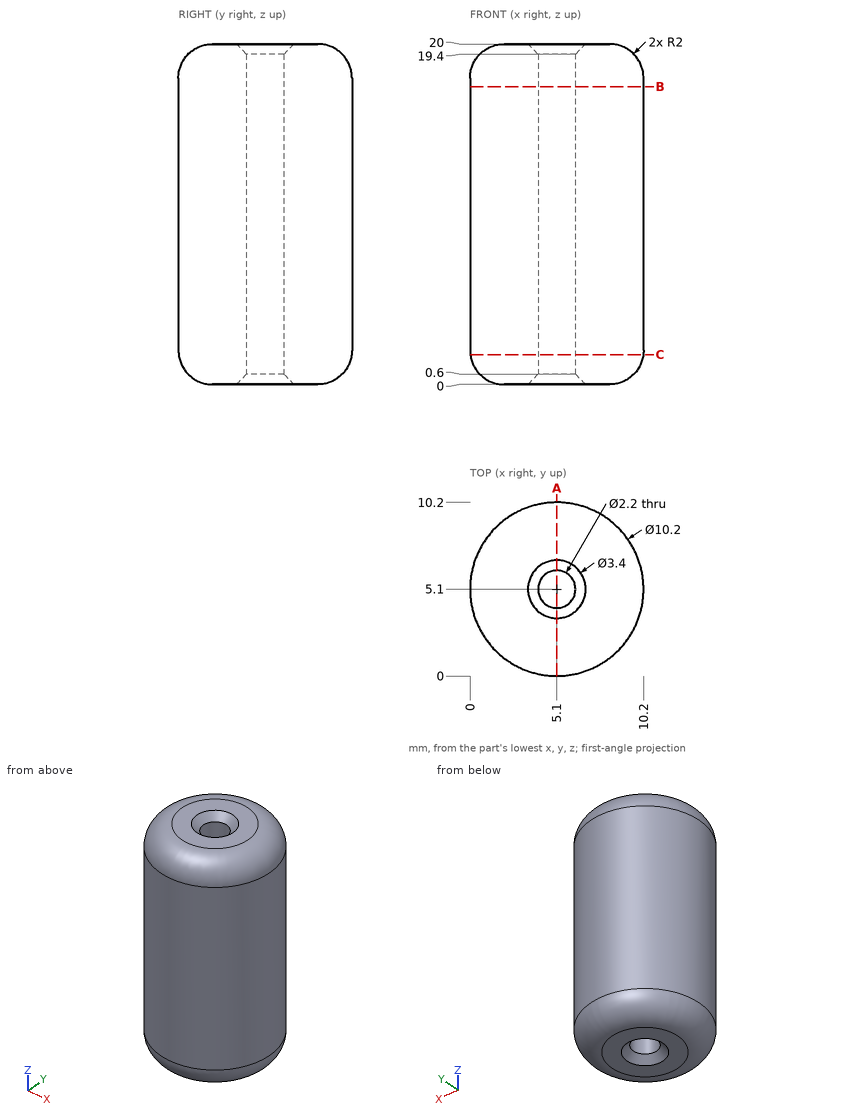
Input: dimensioned drawing with shaded views. Units: mm. Origin: part minimum x, y, z. Round coordinates to 2 decimals unless told otherwise and drop trailing zeros. Order: outer loops, then holes, each group sorted by start corner. A loop starts at its lowest first (then second) coordinate and runs counter-clockwise, first axis right, second up.
1. Pin query (flat end, axial travel): P1, Ø2.5, axis at x = 5.1, y = 5.1, coming from the +Z side; P2, Ø2, axis at x = 5, y = 5.5, coming from the -Z side; P3, Ø2, axis at x = 8, z = 15.5, coming from the +Y side. Return the tip coordinate at first contact, or that it passes through.
The answers:
P1: stops at z = 19.55
P2: stops at z = 0.29
P3: stops at y = 9.83
2. Cut plane B-B, the plane z = 17.5. Output: boundary loops of the cut face in (x, y), then the cut area to 3 significant figures.
The answers:
outline: circle Ø10.2 at (5.1, 5.1); hole circle Ø2.2 at (5.1, 5.1)
area: 77.9 mm2
3. Material intervals for line 1 (Y direction, x = 5.1, z = 15.25); line 2 (X direction, y = 6, z = 16); line 3 (Z direction, x = 2, y = 7.25), sorted ascending.
The answers:
line 1: y = 0 to 4, 6.2 to 10.2
line 2: x = 0.08 to 4.47, 5.73 to 10.12
line 3: z = 0.12 to 19.88
4. Cut plane A-A, the plane x = 5.1. Output: boundary loops of the cut face in (y, z), then the cut area to 3 significant figures.
The answers:
outline: (0, 2) arc R2 ccw to (2, 0) - (3.4, 0) - (4, 0.6) - (4, 19.4) - (3.4, 20) - (2, 20) arc R2 ccw to (0, 18) - close; (6.2, 0.6) - (6.8, 0) - (8.2, 0) arc R2 ccw to (10.2, 2) - (10.2, 18) arc R2 ccw to (8.2, 20) - (6.8, 20) - (6.2, 19.4) - close
area: 156 mm2
5. Cut plane C-C, the plane z = 1.75. Output: boundary loops of the cut face in (x, y).
The answers:
outline: circle Ø10.17 at (5.1, 5.1); hole circle Ø2.2 at (5.1, 5.1)
